Model file for the job. Use its own axes, mm. Face numbers are marked on the shaded views. Coordinates: 2 decimals unless noted, no trailing zeros. Loops run counter-clockwise (first coordinate to the right, second up) from the corner with the lowest first, then second, coordinate; pieces in that order, holes last.
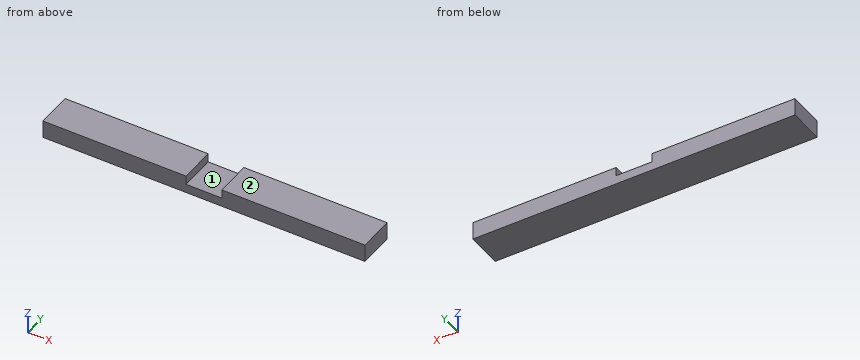
from build123d import *

# Parameters (mm, degrees)
F0_W     = 914.4
F0_H     = 50.8
F1_DEPTH = 50.8
F2_W     = 101.6
F2_H     = 101.6
F3_DEPTH = 25.4


with BuildPart() as f1:
    # F0 (on Front) → F1 (new body, symmetric)
    with BuildSketch(Plane.XZ):
        Rectangle(F0_W, F0_H)
    extrude(amount=F1_DEPTH, both=True)

    # F2 (on face) → F3 (cut)
    with BuildSketch(Plane.XY.offset(25.4)):
        Rectangle(F2_W, F2_H)
    extrude(amount=-F3_DEPTH, mode=Mode.SUBTRACT)


solid = f1.part
Q1. Slice it at B-B (y = 24). List the corners of the cut face in (x, z).
Answers:
outline: (-457.2, -25.4) - (457.2, -25.4) - (457.2, 25.4) - (50.8, 25.4) - (50.8, 0) - (-50.8, 0) - (-50.8, 25.4) - (-457.2, 25.4) - close
Q2. Slice it at A-A (z = 8.5). List the corners of the cut face in (x, y).
Answers:
outline: (-457.2, -50.8) - (-50.8, -50.8) - (-50.8, 50.8) - (-457.2, 50.8) - close; (50.8, -50.8) - (457.2, -50.8) - (457.2, 50.8) - (50.8, 50.8) - close
Q3. Mould opens along X. For the marked faces 1 and 2 say: +X half, -X half, draft (parallel to the pull), parting line (faces both ways), or undercut.
Answers:
face 1: undercut
face 2: draft
Q4. Drill centre line: line 1 (X direction, y = -39, z = 11.5). Where is it in solid material? Low to high.
Answers:
line 1: x = -457.2 to -50.8, 50.8 to 457.2
